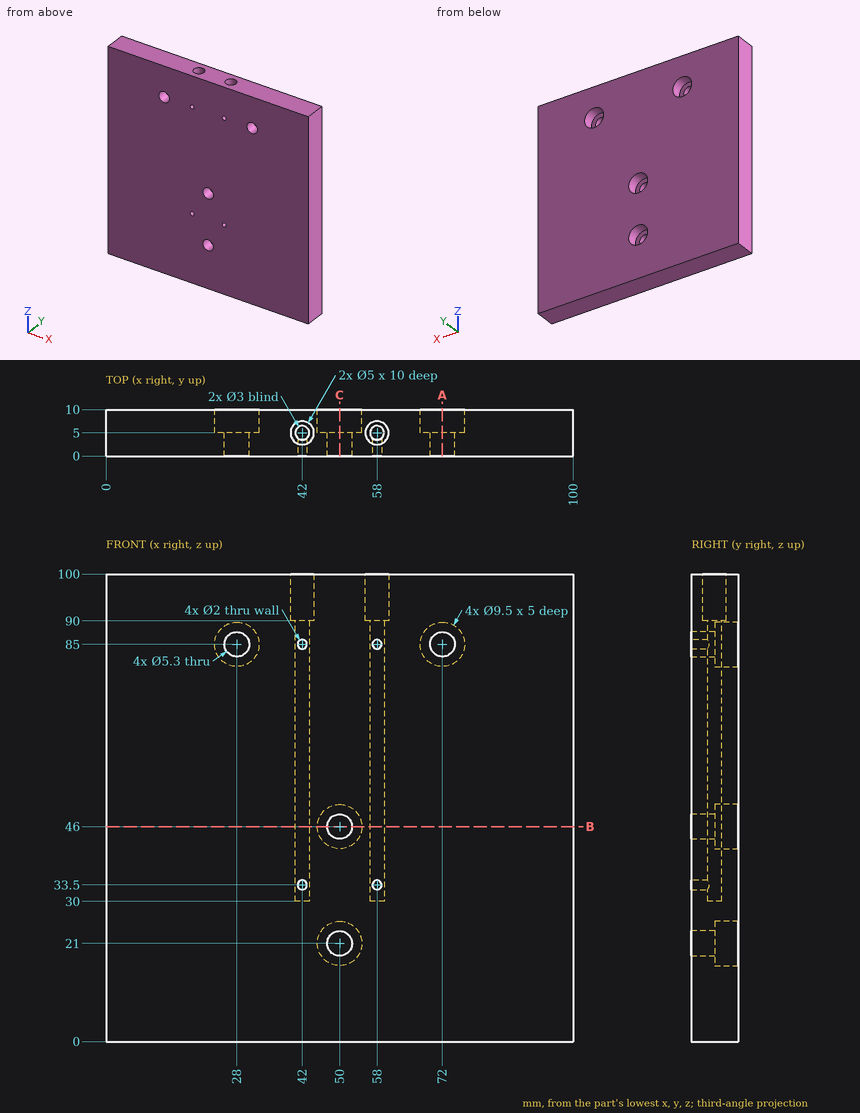
Print and shaded views of the part. All mm, measured from the part's lowest x, y and z. Coordinates: 2 decimals unless noted, no trailing zeros. Loops run counter-clockwise (first coordinate to the right, second up) from the corner with the lowest first, then second, coordinate; pieces in that order, holes last. Notation, with made-up numbers: M 15.5,77 L 31.5,77 A19 ccw 31.5,112 Z; hole C 38.5,-34.5 d7. An arc over 180 degrees is marked long. Use a Markdown table: item, result. Add a question column.
Q1. Cut at C-C (x = 50). Write the cut outline in (y, z).
Q2. Probe L1, parallel to X at y = 1.55, z = 85; L2, parallel to X at y = 8.9, z = 46; L3, parallel to Z at x = 58, y = 1.6. List the from-to ranges inside material, lowest first.
Q3. Cut at A-A (x = 72). Write the cut outline in (y, z).
Q4. Pin check, flat tips, straight feed: P1, Ø4, axis at x = 28, z = 85, coming from the -Y side; P2, Ø2.5, axis at x = 42.5, y = 4.5, coming from the +Z side; P3, Ø7, axis at x = 50, z = 46, coming from the +Y side; P4, Ø1.8, axis at x = 58, z = 85, coming from the -Y side. Stop position of each tip, or through.
Q5. Cut at B-B (z = 46). Write the cut outline in (x, y), and give its area (3 significant figures).
Worked out:
| question | item | result |
|---|---|---|
| 1 | outline | M 0,0 L 10,0 L 10,16.25 L 5,16.25 L 5,18.35 L 0,18.35 Z; M 0,23.65 L 5,23.65 L 5,25.75 L 10,25.75 L 10,41.25 L 5,41.25 L 5,43.35 L 0,43.35 Z; M 0,48.65 L 5,48.65 L 5,50.75 L 10,50.75 L 10,100 L 0,100 Z |
| 2 | L1 | x = 0 to 25.35, 30.65 to 41, 43 to 57, 59 to 69.35, 74.65 to 100 |
| 2 | L2 | x = 0 to 45.25, 54.75 to 100 |
| 2 | L3 | z = 0 to 32.5, 34.5 to 84, 86 to 100 |
| 3 | outline | M 0,0 L 10,0 L 10,80.25 L 5,80.25 L 5,82.35 L 0,82.35 Z; M 0,87.65 L 5,87.65 L 5,89.75 L 10,89.75 L 10,100 L 0,100 Z |
| 4 | P1 | passes through |
| 4 | P2 | stops at z = 90 |
| 4 | P3 | stops at y = 5 |
| 4 | P4 | stops at y = 6.2 |
| 5 | outline | M 0,0 L 47.35,0 L 47.35,5 L 45.25,5 L 45.25,10 L 0,10 Z; M 52.65,0 L 100,0 L 100,10 L 54.75,10 L 54.75,5 L 52.65,5 Z; hole C 42,5 d3; hole C 58,5 d3 |
| 5 | area | 912 mm2 |
